For this review, take the finished solid that the model builds, in its own axes (mm). Face numbers are marked on the shaded views. A direction names the side the tool comes from. Give positions to 0.01 mm unless a question says otherwise; leave off trailing zeros. Write each loop counter-clockwise with the first axis right and the second up, starting at its lowest first coordinate (ties: lowest second). Pieces come first, ordered by that corner, then holes.
Q1. Insertion check: P1, Ø5, axis at x = 42, y = -8.5, coming from the -Z side; P2, Ø1.9, axis at x = 74.38, y = -3.45, coming from the +Z side; P3, Ø1.8, axis at x = -2.59, y = -0.08, coming from the -Z side. Each pin has a flat end and moves straight along its axis. Give the tip position at first contact, or say it passes through.
Q2. Mouldability with a two-part tool opening along X and no side actions: class the marked faces 1, 2, 3 and 4 as released by +X, released by -X, zero draft, split by the parting line, or undercut.
Q3. Machinability: for the marked faces 5, 6 and 7, which of the approach directions +Z, -Z, +X, -X, +Y, -Y give a long, thin tool a straight path to every point of the face, cutting with its end or side? Answer none if there is none.
Q4. We need section C-C (z = 5.5). Write out the cut boundary in (x, y), then the cut area to 3 significant figures.
Q5. We need section B-B (x = 42). Write out the cut boundary in (y, z), then the cut area to 3 significant figures.
Q6. We need section A-A (y = -59.5). Write out the cut boundary in (x, z).
Q7. For line 1 (X direction, y = -39, z = 9.75); line 2 (Y direction, x = 64.5, z = 3); line 3 (Z direction, x = -6.5, y = -85.5), list the stretches that pass through material, from the lowest coordinate up.
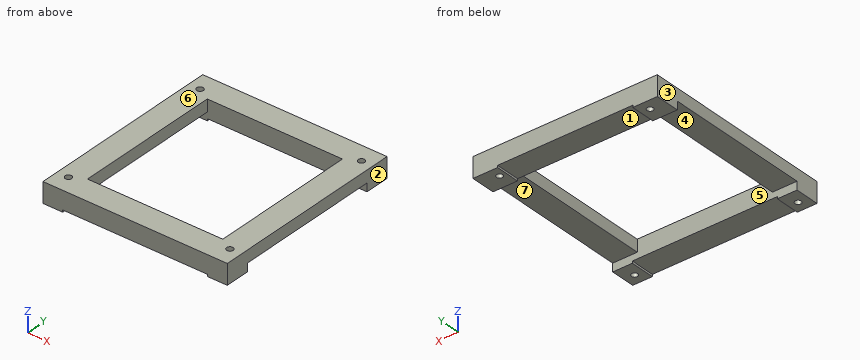
Autodesk Inventor part; units mm, degrees
ref_plane "YZ Plane" through (0, 0, 0) normal (1, 0, 0) x (0, 1, 0)
ref_plane "XZ Plane" through (0, 0, 0) normal (0, 1, 0) x (-1, 0, 0)
ref_plane "XY Plane" through (0, 0, 0) normal (0, 0, 1) x (1, 0, 0)
sketch "Sketch1" plane through (0, 0, 0) normal (0, 0, 1) x (1, 0, 0)
  line L0 (-10.2061, 4.9951) -> (79.9639, 4.9951)
  line L1 (79.9639, 4.9951) -> (79.9639, -90.8899)
  line L2 (79.9639, -90.8899) -> (-10.2061, -90.8899)
  line L3 (-10.2061, -90.8899) -> (-10.2061, 4.9951)
  line L4 (67.9639, -78.8899) -> (1.7939, -78.8899)
  line L5 (67.9639, -78.8899) -> (67.9639, -7.0049)
  line L6 (67.9639, -7.0049) -> (1.7939, -7.0049)
  line L7 (1.7939, -7.0049) -> (1.7939, -78.8899)
  point P0 (0, 0)
  dimension "d0" = 90.17
  dimension "d1" = 95.885
extrude "Extrusion1" add sketch "Sketch1" along normal blind 9.906
sketch "Sketch2" plane through (0, 0, 9.906) normal (0, 0, 1) x (1, 0, 0)
  circle A0 centre (-4.6211, -82.4449) radius 1.6
  circle A1 centre (74.3789, -82.4449) radius 1.6
  circle A2 centre (-4.6211, -3.4499) radius 1.6
  circle A3 centre (74.3789, -3.4499) radius 1.6
  line L0 (79.9639, 4.9951) -> (-10.2061, 4.9951)
  line L1 (-10.2061, -90.8899) -> (79.9639, -90.8899)
  line L2 (79.9639, -90.8899) -> (79.9639, 4.9951)
  line L3 (-10.2061, 4.9951) -> (-10.2061, -90.8899)
  point P0 (0, 0)
  dimension "d18" = 3.2
  dimension "d19" = 3.2
  dimension "d20" = 3.2
  dimension "d21" = 3.2
  dimension "d22" = 8.445
  dimension "d23" = 8.445
  dimension "d24" = 8.445
  dimension "d25" = 8.445
  dimension "d26" = 5.585
  dimension "d27" = 5.585
  dimension "d28" = 5.585
  dimension "d29" = 5.585
extrude "Extrusion2" cut sketch "Sketch2" against normal blind 3.302 contours A0 | A1 | A2 | A3
thread "Thread1"
thread "Thread2"
thread "Thread3"
thread "Thread4"
sketch "Sketch3" plane through (0, 0, 0) normal (0, 0, -1) x (-1, 0, 0)
  circle A0 centre (-71.0739, -0.0849) radius 1.524
  circle A1 centre (5.1261, -85.8099) radius 1.524
  circle A2 centre (-74.8839, -85.8099) radius 1.524
  circle A3 centre (2.5861, -0.0849) radius 1.524
  line L0 (-79.9639, 4.9951) -> (10.2061, 4.9951)
  line L1 (-79.9639, -90.8899) -> (-79.9639, 4.9951)
  line L2 (10.2061, -90.8899) -> (-79.9639, -90.8899)
  line L3 (10.2061, 4.9951) -> (10.2061, -90.8899)
  point P0 (0, 0)
  dimension "d40" = 3.048
  dimension "d41" = 3.048
  dimension "d42" = 3.048
  dimension "d43" = 3.048
  dimension "d45" = 8.89
  dimension "d46" = 90.805
  dimension "d47" = 5.08
  dimension "d48" = 5.08
  dimension "d50" = 85.09
  dimension "d51" = 5.08
  dimension "d52" = 82.55
  dimension "d53" = 90.805
extrude "Extrusion3" cut sketch "Sketch3" against normal blind 3.302 contours A0 | A1 | A2 | A3
sketch "Sketch4" plane through (0, 0, 0) normal (0, 0, -1) x (-1, 0, 0)
  line L0 (-1.7939, -7.0049) -> (-67.9639, -7.0049)
  line L1 (-1.7939, -7.0049) -> (10.2061, -7.0049)
  line L2 (10.2061, 4.9951) -> (10.2061, -90.8899)
  line L3 (-1.7939, -78.8899) -> (10.2061, -78.8899)
  line L4 (-67.9639, -78.8899) -> (-1.7939, -78.8899)
  line L5 (10.2061, -78.8899) -> (-67.9639, -78.8899)
  line L6 (-67.9639, -78.8899) -> (-79.9639, -78.8899)
  line L7 (-79.9639, -90.8899) -> (-79.9639, 4.9951)
  line L8 (-67.9639, -7.0049) -> (-79.9639, -7.0049)
  line L9 (-67.9639, -7.0049) -> (-67.9639, -78.8899)
  line L10 (-67.9639, -7.8922) -> (-67.9639, -78.8899)
  line L11 (-67.9639, -78.8899) -> (-79.9639, -78.8899)
  line L12 (-1.7939, -7.0049) -> (-67.9639, -7.0049)
  line L13 (-79.9639, -7.0049) -> (-1.7939, -7.0049)
  line L14 (-1.7939, -78.8899) -> (-1.7939, -7.0049)
  line L15 (-1.7939, -7.0049) -> (-1.7939, -78.8899)
  line L16 (-1.7939, -78.8899) -> (10.2061, -78.8899)
  point P0 (0, 0)
extrude "Extrusion4" cut sketch "Sketch4" against normal blind 4 contours L1 L2 L3 L14 | L9 L6 L7 L8
sketch "Sketch5" plane through (0, 0, 0) normal (0, 0, -1) x (-1, 0, 0)
  line L0 (-79.9639, 4.9951) -> (10.2061, 4.9951)
  circle A0 centre (-71.0739, -0.0849) radius 1.524
  circle A1 centre (2.5861, -0.0849) radius 1.524
  line L1 (-1.7939, -7.0049) -> (-67.9639, -7.0049)
  line L2 (-1.7939, -7.0049) -> (-1.7939, 4.9951)
  line L3 (-67.9639, -7.0049) -> (-67.9639, 4.9951)
  line L4 (-67.9639, -7.0049) -> (-67.9639, -78.8899)
  line L5 (-67.9639, -78.8899) -> (-67.9639, -90.8899)
  line L6 (10.2061, -90.8899) -> (-79.9639, -90.8899)
  line L7 (-67.9639, -78.8899) -> (-1.7939, -78.8899)
  line L8 (-1.7939, -78.8899) -> (-1.7939, -90.8899)
  point P0 (0, 0)
extrude "Extrusion5" cut sketch "Sketch5" against normal blind 1 contours L7 L8 L6 L5 | L0 L2 L1 L3
sketch "Sketch6" plane through (0, 0, 0) normal (0, 0, -1) x (-1, 0, 0)
  line L0 (0.5761, -90.8899) -> (0.5761, -83.261)
  circle A0 centre (-74.8839, -85.8099) radius 1.524
  circle A1 centre (5.1261, -85.8099) radius 1.524
  line L1 (0.5761, -83.261) -> (0.5761, -78.8899)
  line L2 (10.2061, -78.8899) -> (-1.7939, -78.8899)
  line L3 (-70.3339, -87.0755) -> (-70.3339, -90.8899)
  line L4 (-70.3339, -87.0755) -> (-70.3339, -78.8899)
  line L5 (-67.9639, -78.8899) -> (-79.9639, -78.8899)
  line L6 (10.2061, -90.8899) -> (-79.9639, -90.8899)
  line L7 (-67.9639, -90.8899) -> (-67.9639, -78.8899)
  line L8 (-70.3339, -78.8899) -> (-70.3339, -90.8899)
  line L9 (-1.7939, -90.8899) -> (0.5761, -90.8899)
  line L10 (-67.9639, -78.8899) -> (-1.7939, -78.8899)
  line L11 (0.5761, -78.8899) -> (-1.7939, -78.8899)
  line L12 (-1.7939, -78.8899) -> (-1.7939, -90.8899)
  line L13 (-1.7939, -78.8899) -> (-1.7939, -90.8899)
  point P0 (0, 0)
  dimension "d63" = 4.55
extrude "Extrusion6" cut sketch "Sketch6" against normal blind 1 contours L6 L12 L2 L1 L0 | L6 L3 L4 L5 L7
thread "Thread5"
thread "Thread6"
thread "Thread7"
thread "Thread8"
equation "\"BendRadius\" = Thickness"
equation "\"BendReliefWidth\" = Thickness"
equation "\"BendReliefDepth\" = 0.5 * Thickness"
equation "\"CornerReliefSize\" = 4 * Thickness"
equation "\"MinimumRemnant\" = 2 * Thickness"
equation "\"TransitionRadius\" = BendRadius"
equation "\"JacobiRadiusSize\" = BendRadius"
equation "\"GapSize\" = Thickness"
properties part number "ThomasBracket v2"
Computed:
1. P1: stops at z = 1
1. P2: stops at z = 6.6
1. P3: stops at z = 3.3
2. face 1: undercut
2. face 2: released by +X
2. face 3: released by -X
2. face 4: zero draft
3. face 5: -Z
3. face 6: +Z, +X, -X, +Y, -Y
3. face 7: -Z, +X, -X
4. outline: (-10.21, -90.89) - (79.96, -90.89) - (79.96, 5) - (-10.21, 5) - close; hole (1.79, -78.89) - (67.96, -78.89) - (67.96, -7) - (1.79, -7) - close
4. area: 3,890 mm2
5. outline: (-90.89, 1) - (-78.89, 1) - (-78.89, 9.91) - (-90.89, 9.91) - close; (-7, 1) - (5, 1) - (5, 9.91) - (-7, 9.91) - close
5. area: 214 mm2
6. outline: (-10.21, 4) - (1.79, 4) - (1.79, 9.91) - (-10.21, 9.91) - close; (67.96, 4) - (79.96, 4) - (79.96, 9.91) - (67.96, 9.91) - close
7. line 1: x = -10.21 to 1.79, 67.96 to 79.96
7. line 2: y = -90.89 to -78.89, -7 to 5
7. line 3: z = 3.3 to 9.91
